Read the model definition and answer for the solid it produces. Units are mm, in the model's axes. Coordinates: 2 decimals unless noted, no trailing zeros. Loops run counter-clockwise (first coordinate to the right, second up) from the corner with the lowest first, then second, coordinate; pieces in that order, holes last. Notation, with made-up numbers: M 42.5,84.5 L 79.5,84.5 A27 ccw 79.5,102.5 Z; hole C 28.25,-4.5 d8. An arc over 180 degrees is marked long. Put each result on its own line as item: value.
from build123d import *

# Parameters (mm, degrees)
SKETCH_1_R      = 2.5
EXTRUDE_1_DEPTH = 60
SKETCH_2_R      = 5
EXTRUDE_2_DEPTH = 30
EXTRUDE_START   = 30
SKETCH_3_R      = 5
EXTRUDE_3_DEPTH = 30
FILLET_2_R      = 10
FILLET_3_R      = 1
FILLET_4_R      = 1


with BuildPart() as part:
    # 草圖1 → 填料-伸長1 (new body)
    with BuildSketch(Plane.XY):
        Circle(SKETCH_1_R)
    extrude(amount=EXTRUDE_1_DEPTH)

    # 草圖2 → 填料-伸長2 (add)
    with BuildSketch(Plane.XY.offset(60)):
        Circle(SKETCH_2_R)
    extrude(amount=EXTRUDE_2_DEPTH)

    # 草圖3 → 填料-伸長3 (add)
    with BuildSketch(Plane(origin=(0, 0, 0), x_dir=(-1, 0, 0), z_dir=(0, 0, -1)).offset(EXTRUDE_START)):
        with Locations(Location((0, 0, 0), (0, 0, 180))):
            Circle(SKETCH_3_R)
    extrude(amount=-EXTRUDE_3_DEPTH)

    # 圓角2
    # the kernel refuses this fillet: 10 mm, written as the material it adds along each edge
    with BuildSketch(Plane(origin=(0, 0, 0), x_dir=(1, 0, 0), z_dir=(0, -1, 0))) as fillet_2_piece_1:
        with BuildLine():
            CenterArc((12.5, 6.614378278), FILLET_2_R, 180, 41.409622109)
            Line((2.5, 6.614378278), (2.3, 6.614378278))
            Line((2.3, 6.614378278), (2.3, 0))
            Line((2.3, 0), (2.5, -0.2))
            ThreePointArc((2.5, -0.2), (3.75, -0.2), (4.85, -0.132287566))
            Line((4.85, -0.132287566), (5, 0))
        make_face()
    revolve(axis=Axis((0, 0, 0), (0, 0, 1)))
    with BuildSketch(Plane(origin=(0, 0, 60), x_dir=(1, 0, 0), z_dir=(0, -1, 0))) as fillet_2_piece_2:
        with BuildLine():
            CenterArc((12.5, -6.614378278), FILLET_2_R, 138.590377891, 41.409622109)
            Line((5, 0), (4.85, 0.132287566))
            ThreePointArc((4.85, 0.132287566), (3.75, 0.2), (2.5, 0.2))
            Line((2.5, 0.2), (2.3, 0))
            Line((2.3, 0), (2.3, -6.614378278))
            Line((2.3, -6.614378278), (2.5, -6.614378278))
        make_face()
    revolve(axis=Axis((0, 0, 60), (0, 0, 1)))

    # 圓角3
    fillet_3_edges = [part.edges().sort_by_distance(p)[0] for p in [
        (-5, 0, -30),
        (-5, 0, 90),
    ]]
    fillet(fillet_3_edges, radius=FILLET_3_R)

    # 圓角4
    fillet_4_edges = [part.edges().sort_by_distance(p)[0] for p in [
        (-5, 0, 0),
        (-5, 0, 60),
    ]]
    fillet(fillet_4_edges, radius=FILLET_4_R)


solid = part.part
1) Given pin 1 Ø5 at (y, z) = (3, 61.5) entering from -X; pin 2 Ø4 at (x, z) = (0.5, 26) entering from +Y; pin 3 Ø2 at (y, z) = (0, 11.5) entering from +X, each flat-ended and moving along its own axis, determine where each tip first touches the part or whether it passes through.
Answer list:
pin 1: stops at x = -4.97
pin 2: stops at y = 2.5
pin 3: stops at x = 2.5
2) Find section A-A, the plane z = 76. Write down the section's boundary in (x, y), plus the area to 3 significant figures.
Answer list:
outline: C 0,0 d10
area: 78.5 mm^2
3) Straight lines are drawn through the part: line 1 (Z direction, x = 3, y = 2); line 2 (Y direction, x = -0.25, z = -6.5); line 3 (Z direction, x = 2.25, y = -3). For each, find the intervals that lie inside material, in ascending order. Write a range as [from, to].
Answer list:
line 1: z = [-30, 2.04], [57.96, 90]
line 2: y = [-4.99, 4.99]
line 3: z = [-30, 1.77], [58.23, 90]
4) Find section B-B, the plane z = 44. Write down the section's boundary in (x, y), plus the area to 3 significant figures.
Answer list:
outline: C 0,0 d5
area: 19.6 mm^2
5) Determine the mould class of faces 1 (the cylindrical face through (4.77, 1.5, 74.48)), 2 (the flat face through (0, 0, 90)), 3 (the cylindrical face through (-0.54, -2.44, 29.67)) for opening direction Z: released by +Z, released by -Z, zero draft, split by the parting line, or undercut.
Answer list:
face 1: zero draft
face 2: released by +Z
face 3: undercut
